Geometry check sheet. Reference: drawing and pictorial views, mm from the part's lowest x, y, z. A direction names the side the tool comes from. Round coordinates to 2 decimals unless told otherwise and drop trailing zeros. Order: outer loops, then holes, each group sorted by start corner. A loop starts at its lowest first (then second) coordinate and runs counter-clockwise, first axis right, second up. Notation, with made-up numbers: (-9, 61) -> (16, 61) arc R21 cw to (16, 75) -> close; hole circle Ø5 at (55.5, 53.5). An arc over 180 degrees is marked (long way). Put each result on its own line as item: value.
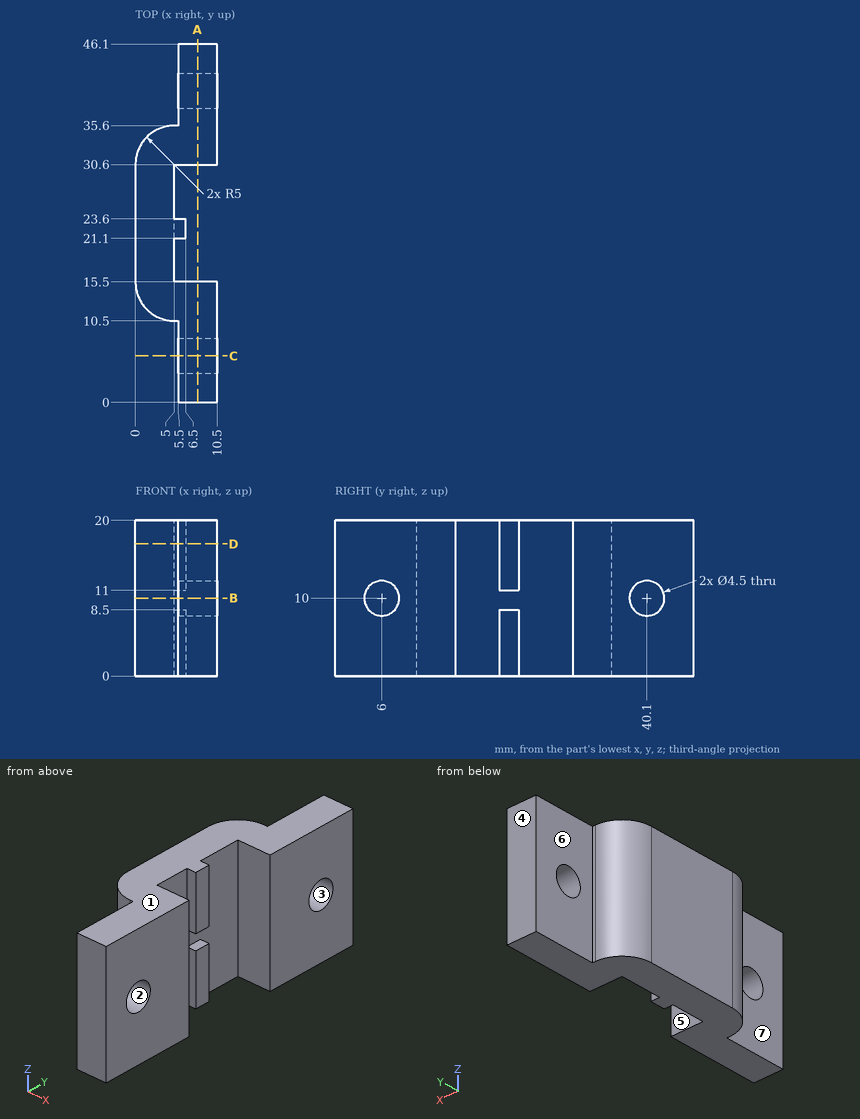
Item 1: Depth check by flat-ended pin: pin 1 Ø2 at (y, z) = (21.5, 16) entering from +X; pin 2 Ø1.5 at (x, y) = (7.5, 18.5) entering from +Z; pin 3 Ø3 at (x, z) = (1.5, 9) entering from -Y. Enter the tip coordinate at first touch or a pass-through.
Geometry check:
pin 1: x = 6.5
pin 2: through
pin 3: y = 10.92
Item 2: Sectioned sample at D-D, the plane z = 17. Record the boundary of the cut face in (x, y), then the cut area to 3 significant figures.
Geometry check:
outline: (0, 15.5) arc R5 ccw to (5, 10.5) -> (5.5, 10.5) -> (5.5, 0) -> (10.5, 0) -> (10.5, 15.5) -> (5, 15.5) -> (5, 21.1) -> (6.5, 21.1) -> (6.5, 23.6) -> (5, 23.6) -> (5, 30.6) -> (10.5, 30.6) -> (10.5, 46.1) -> (5.5, 46.1) -> (5.5, 35.6) -> (5, 35.6) arc R5 ccw to (0, 30.6) -> close
area: 279 mm2
Item 3: Sectioned sample at B-B, the plane z = 10. Record the boundary of the cut face in (x, y), then the cut area to 3 significant figures.
Geometry check:
outline: (0, 15.5) arc R5 ccw to (5, 10.5) -> (5.5, 10.5) -> (5.5, 8.25) -> (10.5, 8.25) -> (10.5, 15.5) -> (5, 15.5) -> (5, 30.6) -> (10.5, 30.6) -> (10.5, 37.85) -> (5.5, 37.85) -> (5.5, 35.6) -> (5, 35.6) arc R5 ccw to (0, 30.6) -> close; (5.5, 0) -> (10.5, 0) -> (10.5, 3.75) -> (5.5, 3.75) -> close; (5.5, 42.35) -> (10.5, 42.35) -> (10.5, 46.1) -> (5.5, 46.1) -> close
area: 230 mm2
Item 4: Sectioned sample at C-C, the plane y = 6. Record the boundary of the cut face in (x, z).
Geometry check:
outline: (5.5, 0) -> (10.5, 0) -> (10.5, 7.75) -> (5.5, 7.75) -> close; (5.5, 12.25) -> (10.5, 12.25) -> (10.5, 20) -> (5.5, 20) -> close
Item 5: Sectioned sample at A-A, the plane x = 8. Record the boundary of the cut face in (y, z).
Geometry check:
outline: (0, 0) -> (15.5, 0) -> (15.5, 20) -> (0, 20) -> close; (30.6, 0) -> (46.1, 0) -> (46.1, 20) -> (30.6, 20) -> close; hole circle Ø4.5 at (6, 10); hole circle Ø4.5 at (40.1, 10)
Item 6: Release check for a two-part mould opening along Z. For the marked faces 1, 2, 3 and 4 record: pulls with the +Z half, pulls with the -Z half, needs draft (parallel to the pull), parting line crosses it, or undercut.
Geometry check:
face 1: pulls with the +Z half
face 2: undercut
face 3: undercut
face 4: needs draft
Item 7: Tool access check on the marked faces 5, 6 and 7. Record the directions out of +Z, -Z, +X, -X, +Y, -Y that give a thin tool (end or side, any length) a straight path to the whole face; none if there is none.
Geometry check:
face 5: +Z, -Z, +X
face 6: +Z, -Z, -X, +Y
face 7: +Z, -Z, -X, -Y
Item 8: Material ranges on line 1 along Y through (x, z) = (5.75, 4.5); line 2 along Y through (x, z) = (8.45, 10); line 3 along Y through (x, z) = (9.5, 6.25), recorded low to high.
Geometry check:
line 1: 0 to 15.5, 21.1 to 23.6, 30.6 to 46.1
line 2: 0 to 3.75, 8.25 to 15.5, 30.6 to 37.85, 42.35 to 46.1
line 3: 0 to 15.5, 30.6 to 46.1
